For this review, take the finished solid that the model builds, in its own axes (mm). A direction names the side the tool comes from. Coordinates: 2 decimals unless noted, no trailing zeros. Loops run counter-clockwise (first coordinate to the right, second up) from the corner with the lowest first, then second, coordinate; pieces in that order, holes last. Notation, with made-up numbers: (20, 73) - (58, 73) arc R21 cw to (58, 82) - close; hole circle Ø6 at (-26, -30.5). An arc over 180 degrees is marked (long way). One line per item, written item: value. Start each with the question number.
1. Insertion check: pin 1 (4.5 mm diameter, centred on y = 15.5, z = 38, fed in from +X); pin 2 (2.5 mm diameter, centred on x = 66.5, z = 2.5, fed in from +Y); pin 3 (2.5 mm diameter, centred on y = -3, z = -2.5, fed in from -X). Each pin has a flat end and moves straight along its axis. Give the tip position at first contact, or say it passes through.
2. Take a section at B-B, the plane z = -4. State the section outline as (x, y) points, and give its area (3 significant figures).
3. Take a section at C-C, the plane x = 79.5. State the section outline as (y, z) points.
4. Take a section at A-A, the plane z = 21. State the section outline as (x, y) points.
5. To check wall thickness, follow line 1 (X direction, y = -3.4, z = 45.85); line 2 (X direction, y = -3.45, z = -4); line 3 (X direction, y = 22, z = 45.85). State the ranges of each line that lie inside material, in increasing order. Write a range as from..to.
6. For faces 1 (the face through (99, -1, 0)), 2 (the face through (48.5, 10, 46)), 3 (the face through (95, -3, 0)), 4 (the face through (67, -2, 5)), list the 3-axis set-ups (+Z, -Z, +X, -X, +Y, -Y) from which the entire face can be reached by the end or side of a thin tool; tool diameter is ignored.
7. Take a section at D-D, the plane y = 22.25. State the section outline as (x, z) points.
```python
from build123d import *

# Parameters (mm, degrees)
BOSS_EXTRUDE1_DEPTH = 24.5
SKETCH2_W           = 103
SKETCH2_H           = 41.85
BOSS_EXTRUDE2_DEPTH = 5
SKETCH3_W           = 46.5
SKETCH3_H           = 27.85
CUT_EXTRUDE1_DEPTH  = 26
SKETCH7_W           = 8
SKETCH7_H           = 3
BOSS_EXTRUDE3_DEPTH = 8
SKETCH8_R           = 2.5
CUT_EXTRUDE2_DEPTH  = 8
SKETCH9_W           = 8
SKETCH9_H           = 3
BOSS_EXTRUDE4_DEPTH = 8
SKETCH10_R          = 2.5
CUT_EXTRUDE3_DEPTH  = 8
SKETCH12_W          = 11.5
SKETCH12_H          = 5
CUT_EXTRUDE4_DEPTH  = 8
SKETCH14_W          = 8
SKETCH14_H          = 3
BOSS_EXTRUDE5_DEPTH = 8
SKETCH15_R          = 2.5
CUT_EXTRUDE5_DEPTH  = 8
SKETCH16_W          = 8
SKETCH16_H          = 29.5
BOSS_EXTRUDE6_DEPTH = 8
SKETCH17_W          = 8
SKETCH17_H          = 29.5
BOSS_EXTRUDE7_DEPTH = 8
SKETCH18_R          = 2
CUT_EXTRUDE6_DEPTH  = 10


with BuildPart() as part:
    # Sketch1 → Boss-Extrude1 (new body)
    with BuildSketch(Plane(origin=(0, 0, 0), x_dir=(1, 0, 0), z_dir=(0, 1, 0))):
        Polygon((0, 0), (51.5, 0), (51.5, -5), (5, -5), (5, -36.85), (51.5, -36.85), (51.5, -32.85), (56.5, -32.85), (56.5, -41.85), (0, -41.85), align=None)
    extrude(amount=BOSS_EXTRUDE1_DEPTH)

    # Sketch2 → Boss-Extrude2 (add)
    with BuildSketch(Plane.XZ):
        with Locations((51.5, 20.925)):
            Rectangle(SKETCH2_W, SKETCH2_H)
    extrude(amount=BOSS_EXTRUDE2_DEPTH)

    # Sketch3 → Cut-Extrude1 (cut)
    with BuildSketch(Plane(origin=(0, 0, 0), x_dir=(1, 0, 0), z_dir=(0, 1, 0))):
        with Locations((74.75, -18.925)):
            Rectangle(SKETCH3_W, SKETCH3_H)
    extrude(amount=-CUT_EXTRUDE1_DEPTH, mode=Mode.SUBTRACT)

    # Sketch7 → Boss-Extrude3 (add)
    with BuildSketch(Plane.XY.offset(41.85)):
        with Locations((4, -3.5)):
            Rectangle(SKETCH7_W, SKETCH7_H)
    extrude(amount=BOSS_EXTRUDE3_DEPTH)

    # Sketch8 → Cut-Extrude2 (cut)
    with BuildSketch(Plane(origin=(0, -2, 0), x_dir=(1, 0, 0), z_dir=(0, 1, 0))):
        with Locations(Location((4, -45.85, 0), (0, 0, 270))):
            Circle(SKETCH8_R)
    extrude(amount=-CUT_EXTRUDE2_DEPTH, mode=Mode.SUBTRACT)

    # Sketch9 → Boss-Extrude4 (add)
    with BuildSketch(Plane(origin=(0, 0, 0), x_dir=(-1, 0, 0), z_dir=(0, 0, -1))):
        with Locations((-99, -3.5)):
            Rectangle(SKETCH9_W, SKETCH9_H)
    extrude(amount=BOSS_EXTRUDE4_DEPTH)

    # Sketch10 → Cut-Extrude3 (cut)
    with BuildSketch(Plane(origin=(0, -2, 0), x_dir=(1, 0, 0), z_dir=(0, 1, 0))):
        with Locations(Location((99, 3.996680608, 0), (0, 0, 270))):
            Circle(SKETCH10_R)
    extrude(amount=-CUT_EXTRUDE3_DEPTH, mode=Mode.SUBTRACT)

    # Sketch12 → Cut-Extrude4 (cut)
    with BuildSketch(Plane(origin=(0, 0, 0), x_dir=(1, 0, 0), z_dir=(0, 1, 0))):
        with Locations((89.25, -2.5)):
            Rectangle(SKETCH12_W, SKETCH12_H)
    extrude(amount=-CUT_EXTRUDE4_DEPTH, mode=Mode.SUBTRACT)

    # Sketch14 → Boss-Extrude5 (add)
    with BuildSketch(Plane(origin=(0, 0, 0), x_dir=(-1, 0, 0), z_dir=(0, 0, -1))):
        with Locations((-79.5, -3.5)):
            Rectangle(SKETCH14_W, SKETCH14_H)
    extrude(amount=BOSS_EXTRUDE5_DEPTH)

    # Sketch15 → Cut-Extrude5 (cut)
    with BuildSketch(Plane(origin=(0, -2, 0), x_dir=(1, 0, 0), z_dir=(0, 1, 0))):
        with Locations(Location((79.5, 4, 0), (0, 0, 270))):
            Circle(SKETCH15_R)
    extrude(amount=-CUT_EXTRUDE5_DEPTH, mode=Mode.SUBTRACT)

    # Sketch16 → Boss-Extrude6 (add)
    with BuildSketch(Plane(origin=(0, 0, 0), x_dir=(-1, 0, 0), z_dir=(0, 0, -1))):
        with Locations((-44.5, 9.75)):
            Rectangle(SKETCH16_W, SKETCH16_H)
    extrude(amount=BOSS_EXTRUDE6_DEPTH)

    # Sketch17 → Boss-Extrude7 (add)
    with BuildSketch(Plane.XY.offset(41.85)):
        with Locations((44.5, 9.75)):
            Rectangle(SKETCH17_W, SKETCH17_H)
    extrude(amount=BOSS_EXTRUDE7_DEPTH)

    # Sketch18 → Cut-Extrude6 (cut)
    with BuildSketch(Plane(origin=(0, 24.5, 0), x_dir=(1, 0, 0), z_dir=(0, 1, 0))):
        with Locations(Location((44.5, 4, 0), (0, 0, 270))):
            Circle(SKETCH18_R)
        with Locations(Location((44.5, -45.85, 0), (0, 0, 270))):
            Circle(SKETCH18_R)
    extrude(amount=-CUT_EXTRUDE6_DEPTH, mode=Mode.SUBTRACT)


solid = part.part
```
Solutions:
1. pin 1: x = 56.5
1. pin 2: y = 0
1. pin 3: x = 40.5
2. outline: (40.5, -5) - (48.5, -5) - (48.5, 24.5) - (46.5, 24.5) - (46.5, 14.5) - (42.5, 14.5) - (42.5, 24.5) - (40.5, 24.5) - close; (75.5, -5) - (77, -5) - (77, -2) - (75.5, -2) - close; (82, -5) - (83.5, -5) - (83.5, -2) - (82, -2) - close; (95, -5) - (96.5, -5) - (96.5, -2) - (95, -2) - close; (101.5, -5) - (103, -5) - (103, -2) - (101.5, -2) - close
2. area: 214 mm2
3. outline: (-5, -8) - (-2, -8) - (-2, -6.5) - (-5, -6.5) - close; (-5, -1.5) - (-2, -1.5) - (-2, 0) - (0, 0) - (0, 5) - (-5, 5) - close; (-5, 32.85) - (0, 32.85) - (0, 41.85) - (-5, 41.85) - close
4. outline: (0, -5) - (51.5, -5) - (51.5, 0) - (5, 0) - (5, 24.5) - (0, 24.5) - close; (98, -5) - (103, -5) - (103, 0) - (98, 0) - close
5. line 1: 0..1.5, 6.5..8, 40.5..48.5
5. line 2: 40.5..48.5, 75.5..77, 82..83.5, 95..96.5, 101.5..103
5. line 3: 40.5..42.5, 46.5..48.5
6. face 1: -Z, +X, +Y
6. face 2: +Z, +X, +Y, -Y
6. face 3: -Z, +Y, -Y
6. face 4: +Y, -Y
7. outline: (0, 0) - (40.5, 0) - (40.5, -8) - (48.5, -8) - (48.5, 0) - (51.5, 0) - (51.5, 5) - (5, 5) - (5, 36.85) - (51.5, 36.85) - (51.5, 32.85) - (56.5, 32.85) - (56.5, 41.85) - (48.5, 41.85) - (48.5, 49.85) - (40.5, 49.85) - (40.5, 41.85) - (0, 41.85) - close; hole circle Ø4 at (44.5, -4); hole circle Ø4 at (44.5, 45.85)
